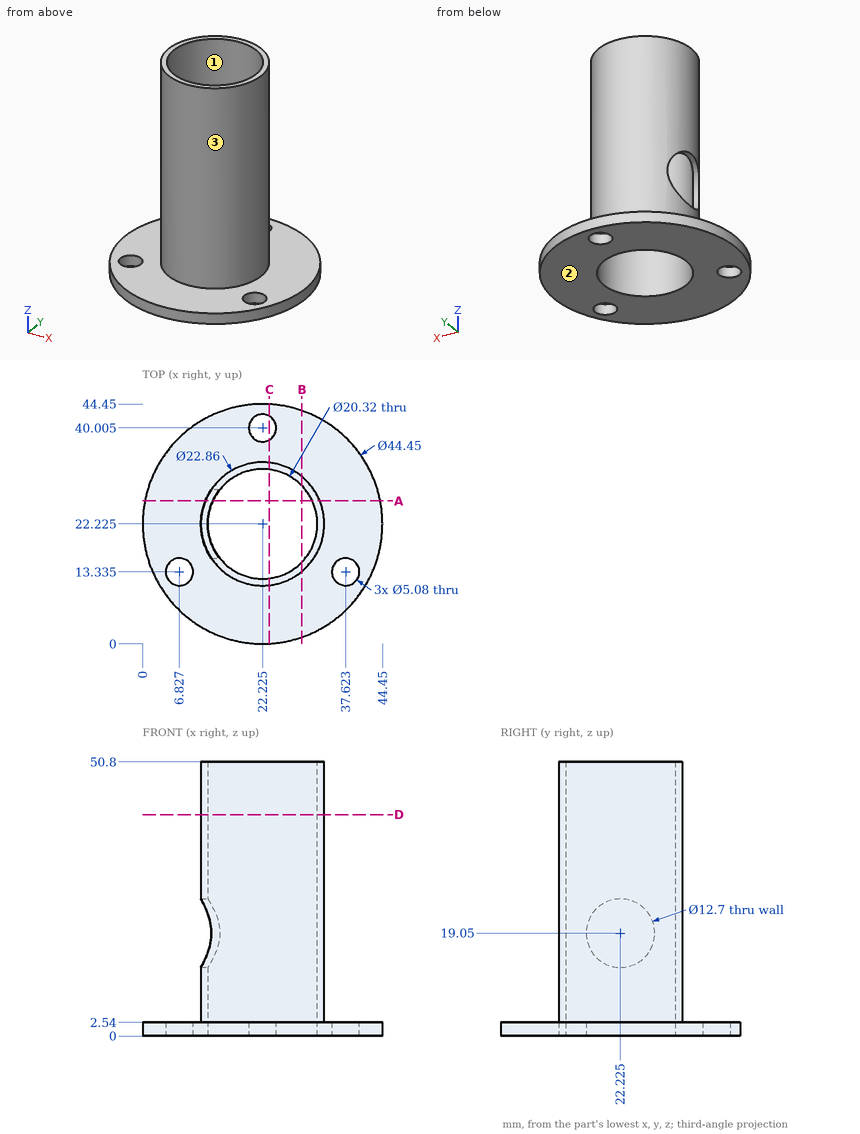
Verification items for this drawing (mm, ordinates from the low corner). Give positions to 0.01 mm unless a question says otherwise; leave off trailing zeros. Write each loop counter-clockwise with the first axis right and the second up, starting at its lowest first coordinate (ties: lowest second). Pieces come first, ordered by that corner, then holes. Notation, with made-up numbers: (44, 17) -> (68, 17) arc R13 cw to (68, 39) -> close; hole circle Ø9 at (-31, 23.5). An arc over 180 degrees is marked (long way). Use CSV: the item, a comma, the result in double quotes. Start each with the question number.
Q1. Depth check by flat-ended pin: P1, Ø12, axis at x = 30.5, z = 23.5, coming from the +Y side; P2, Ø12, axis at x = 25.5, y = 34.5, coming from the +Z side; P3, Ø3, axis at y = 25.5, z = 9, coming from the +X side; P4, Ø11.5, axis at y = 22.225, z = 19.05, coming from the -X side. Enter the tip coordinate at first touch or a pass-through.
Q2. Cross-section at A-A on y = 26.5. Enter the section's corners in (x, z) (1 decimal).
Q3. Cross-section at B-B on x = 29.5. Enter the section's corners in (y, z).
Q4. Scan lines: line 1 along X through (y, z) = (22.5, 35); line 2 along Z through (x, y) = (13.5, 8); line 3 along Y through (x, z) = (16, 47). Record each from-to range of solid material in increasing order.
Q5. Cross-section at C-C on x = 23.5. Enter the section's corners in (y, z), and give its area (3 significant figures).
Q6. Release check for a two-part mould opening along X. For the marked faces 1, 2 and 3 record: +X half, -X half, draft (parallel to the pull), parting line (faces both ways), or undercut.
Q7. Cross-section at D-D on z = 41. Enter the section's corners in (x, y) (3 decimals).
Working result:
1,P1,"stops at y = 33.43"
1,P2,"stops at z = 50.8"
1,P3,"stops at x = 33.52"
1,P4,"stops at x = 30.6"
2,outline,"(0.4, 0) -> (13, 0) -> (13, 14.4) -> (11.6, 14.4) -> (11.6, 2.5) -> (0.4, 2.5) -> close; (11.6, 23.7) -> (13, 23.7) -> (13, 50.8) -> (11.6, 50.8) -> close; (31.4, 0) -> (44, 0) -> (44, 2.5) -> (32.8, 2.5) -> (32.8, 50.8) -> (31.4, 50.8) -> close"
3,outline,"(1.22, 0) -> (15.13, 0) -> (15.13, 50.8) -> (13.41, 50.8) -> (13.41, 2.54) -> (1.22, 2.54) -> close; (29.32, 0) -> (43.23, 0) -> (43.23, 2.54) -> (31.04, 2.54) -> (31.04, 50.8) -> (29.32, 50.8) -> close"
4,line 1,"x = 10.8 to 12.07, 32.38 to 33.65"
4,line 2,"z = 0 to 2.54"
4,line 3,"y = 12.64 to 14.2, 30.25 to 31.81"
5,outline,"(0.04, 0) -> (12.15, 0) -> (12.15, 50.8) -> (10.87, 50.8) -> (10.87, 2.54) -> (0.04, 2.54) -> close; (32.3, 0) -> (37.81, 0) -> (37.81, 2.54) -> (33.58, 2.54) -> (33.58, 50.8) -> (32.3, 50.8) -> close; (42.2, 0) -> (44.41, 0) -> (44.41, 2.54) -> (42.2, 2.54) -> close"
5,area,"174 mm^2"
6,face 1,"undercut"
6,face 2,"draft"
6,face 3,"parting line"
7,outline,"circle Ø22.86 at (22.225, 22.225); hole circle Ø20.32 at (22.225, 22.225)"
